from build123d import *

# Parameters (mm, degrees)
F0_W     = 20
F0_H     = 3
F1_DEPTH = 40
F2_W     = 21.25
F2_H     = 5
F3_DEPTH = 50


with BuildPart() as f1:
    # F0 (on Front) → F1 (new body)
    with BuildSketch(Plane.XZ):
        with Locations((-17.720056, 19.5)):
            Rectangle(F0_W, F0_H)
        Polygon((-27.720056, 18), (-27.720056, 21), (-32.048252, 21), (-32.048252, 17), (-32.048252, 3.254739), (-32.00801, 3.254739), (-27.720056, 3.254739), align=None)
        with BuildLine():
            Line((-32.048252, 17), (-32.048252, 21))
            ThreePointArc((-32.048252, 21), (-42.326909, 26.807327), (-42.65698, 38.608466))
            ThreePointArc((-42.65698, 38.608466), (-40.843318, 42.27556), (-44.92868, 42.491816))
            ThreePointArc((-44.92868, 42.491816), (-46.328817, 25.784359), (-32.048252, 17))
        make_face()
        with BuildLine():
            ThreePointArc((-22.679552, 0), (-26.827174, -0.892883), (-27.720056, 3.254739))
            Line((-27.720056, 3.254739), (-32.00801, 3.254739))
            ThreePointArc((-32.00801, 3.254739), (-28.422472, -4.58668), (-19.947428, -3))
            Line((-19.947428, -3), (-22.679552, -3))
            Line((-22.679552, -3), (-22.679552, 0))
        make_face()
        Polygon((-7.813289, 0), (-22.679552, 0), (-22.679552, -3), (-19.947428, -3), (-7.813289, -3), align=None)
    extrude(amount=F1_DEPTH)

    # F2 (on Top) → F3 (cut)
    with BuildSketch(Plane.XY):
        with Locations((-45.717653, -10)):
            Rectangle(F2_W, F2_H)
        with Locations((-45.717653, -30)):
            Rectangle(F2_W, F2_H)
    extrude(amount=F3_DEPTH, mode=Mode.SUBTRACT)


solid = f1.part
Design review of the part built by this model. Coordinates are the model's own, in mm. A direction names the side the tool comes from. Give positions to 0.01 mm unless a question says otherwise; leave off trailing zeros. Loops run counter-clockwise (first coordinate to the right, second up) from the corner with the lowest first, then second, coordinate; pieces in that order, holes last. Notation, with made-up numbers: (66, 78.5) -> (125, 78.5) arc R16 ccw to (125, 94.5) -> close; hole circle Ø11 at (63, -6). An arc over 180 degrees is marked (long way). One line per question, with ' | ' between items. Start each with the question number.
(1) We need section C-C (y = -30.5). State the section outline as (x, z) points, and give its area (3 significant figures).
(2) Draft analysis for pull direction Z (two halves, no side actions). For faces 1 (the face through (-20, -20, 21)), 2 (the face through (-18, -20, 18)), 3 (the face through (-45, -27.5, 30)), state which applies: +Z half, -Z half, draft (parallel to the pull), parting line (faces both ways), or undercut.
(3) For faces 4 (the face through (-35.093, -10, 19)), 5 (the face through (-15, -20, 0)), 6 (the face through (-7.813, -20, -2)), 7 (the face through (-32.048, -20, 10)), list the 3-axis set-ups (+Z, -Z, +X, -X, +Y, -Y) from which the entire face can be reached by the end or side of a thin tool; tool diameter is ignored.
(4) We need section A-A (x = -18). State the section outline as (y, z) points.
(5) Insertion check: P1, Ø6, axis at x = -18.5, y = -21, coming from the -Z side (3 decimals); P2, Ø4, axis at x = -29, y = -12, coming from the +Z side; P3, Ø4.5, axis at y = -9.5, z = 20, coming from the -X side. Each pin has a flat end and moves straight along its axis. Give the tip position at first contact, or say it passes through.
(6) We need section D-D (z = 33). State the section outline as (x, y) points.
(7) For line 1 (Z direction, x = -13.5, y = -38); line 2 (Z direction, x = -25.5, y = -30); line 3 (X direction, y = -36.5, z = -1.5), list the stretches that pass through material, from the lowest coordinate up.
(8) We need section B-B (z = 25.5). State the section outline as (x, y) points.
The answers:
1) outline: (-35.09, 17.29) arc R16 ccw to (-32.05, 17) -> (-32.05, 3.25) -> (-32.01, 3.25) arc R7 ccw to (-19.95, -3) -> (-7.81, -3) -> (-7.81, 0) -> (-22.68, 0) arc R3 cw to (-27.72, 3.25) -> (-27.72, 18) -> (-7.72, 18) -> (-7.72, 21) -> (-32.05, 21) arc R12 cw to (-35.09, 21.39) -> close | area: 246 mm^2
2) face 1: +Z half | face 2: undercut | face 3: draft
3) face 4: +Z, -Z, -X | face 5: +X, +Y, -Y | face 6: -Z, +X, +Y, -Y | face 7: -X, +Y, -Y
4) outline: (-40, -3) -> (0, -3) -> (0, 0) -> (-40, 0) -> close; (-40, 18) -> (0, 18) -> (0, 21) -> (-40, 21) -> close
5) P1: stops at z = -4.315 | P2: stops at z = 21 | P3: stops at x = -42.67
6) outline: (-48.05, -40) -> (-44.05, -40) -> (-44.05, -32.5) -> (-48.05, -32.5) -> close; (-48.05, -27.5) -> (-44.05, -27.5) -> (-44.05, -12.5) -> (-48.05, -12.5) -> close; (-48.05, -7.5) -> (-44.05, -7.5) -> (-44.05, 0) -> (-48.05, 0) -> close
7) line 1: z = -3 to 0, 18 to 21 | line 2: z = -5.37 to -1.36, 18 to 21 | line 3: x = -31.46 to -7.81
8) outline: (-46.18, -40) -> (-41.42, -40) -> (-41.42, -32.5) -> (-46.18, -32.5) -> close; (-46.18, -27.5) -> (-41.42, -27.5) -> (-41.42, -12.5) -> (-46.18, -12.5) -> close; (-46.18, -7.5) -> (-41.42, -7.5) -> (-41.42, 0) -> (-46.18, 0) -> close
